Print and shaded views of the part. All mm, measured from the part's lowest x, y and z. Round coordinates to 2 decimals unless told otherwise and drop trailing zeros. Order: outer loops, then holes, each group sorted by start corner. A loop starts at its lowest first (then second) coordinate and runs counter-clockwise, first axis right, second up. Notation, with made-up numbers: (-14.75, 56) - (13.25, 56) arc R34 cw to (13.25, 90) - close; hole circle Ø1 at (12.5, 9). An arc over 180 degrees is marked (long way). Write item = value, one per line.
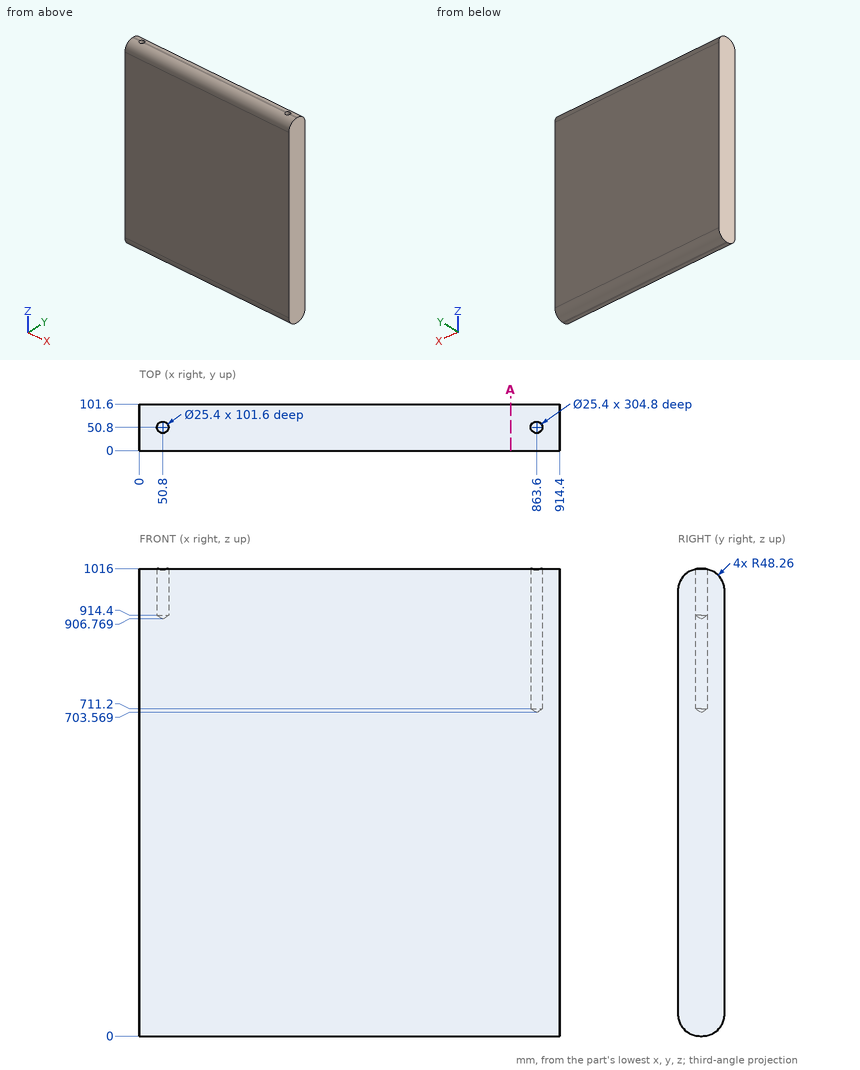
(1) Drop flat-ended pins along their axis: pin 1 (15 mm diameter, centred on x = 863.6, y = 50.8, fed in from +Z); pin 2 (8 mm diameter, centred on x = 441.5, y = 72, fed in from -Z); pin 3 (20.5 mm diameter, centred on x = 50.8, y = 50.8, fed in from +Z). Give the stop position or say it passes through.
Solved:
pin_1 = 708.08
pin_2 = 2.28
pin_3 = 912.93
(2) Band-saw the part on A-A on x = 807. List the corners of the cut face in (y, z).
Solved:
outline = (0, 48.26) arc R48.26 ccw to (48.26, 0) - (53.34, 0) arc R48.26 ccw to (101.6, 48.26) - (101.6, 967.74) arc R48.26 ccw to (53.34, 1016) - (48.26, 1016) arc R48.26 ccw to (0, 967.74) - close
(3) Probe line 1 along X through (y, z) = (50, 947); line 2 along Y through (x, z) = (50, 952); line 3 along X through (y, z) = (54.5, 932). List the from-to ranges inside material, lowest first.
Solved:
line_1 = 0 to 38.13, 63.47 to 850.93, 876.27 to 914.4
line_2 = 0 to 38.13, 63.47 to 101.6
line_3 = 0 to 38.65, 62.95 to 851.45, 875.75 to 914.4
